from build123d import *

# Parameters (mm, degrees)
SKETCH1_W           = 160
SKETCH1_H           = 140
BOSS_EXTRUDE1_DEPTH = 16
SKETCH2_R           = 6.5
CUT_EXTRUDE1_DEPTH  = 11
SKETCH3_R           = 3
CUT_EXTRUDE2_DEPTH  = 214.20412754


with BuildPart() as part:
    # Sketch1 → Boss-Extrude1 (new body)
    with BuildSketch(Plane.XY):
        with Locations((-80, -70)):
            Rectangle(SKETCH1_W, SKETCH1_H)
    extrude(amount=BOSS_EXTRUDE1_DEPTH)

    # Sketch2 → Cut-Extrude1 (cut)
    with BuildSketch(Plane.XY.offset(16)):
        with Locations((-131.336336798, -99.63904787)):
            Circle(SKETCH2_R)
        with Locations((-80, -10.721904261)):
            Circle(SKETCH2_R)
        with Locations((-28.663663202, -99.63904787)):
            Circle(SKETCH2_R)
    extrude(amount=-CUT_EXTRUDE1_DEPTH, mode=Mode.SUBTRACT)

    # Sketch3 → Cut-Extrude2 (cut, through all)
    with BuildSketch(Plane.XY.offset(16)):
        with Locations((-18, -43)):
            Circle(SKETCH3_R)
        with Locations((-102, -43)):
            Circle(SKETCH3_R)
    extrude(amount=-CUT_EXTRUDE2_DEPTH, mode=Mode.SUBTRACT)


solid = part.part
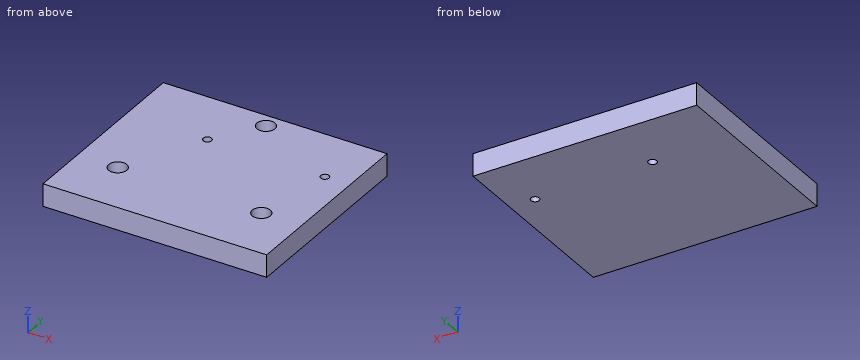
Design review of the part built by this model. Coordinates are the model's own, in mm. Round coordinates to 2 decimals unless told otherwise and drop trailing zeros. Write each loop counter-clockwise with the first axis right and the second up, starting at its lowest first coordinate (ties: lowest second). Pieces come first, ordered by that corner, then holes. Notation, with made-up numbers: (-13.5, 43) -> (40.5, 43) arc R6 ccw to (40.5, 53) -> close; hole circle Ø7 at (19.25, 6.25). An arc over 180 degrees is marked (long way). One line per item, written item: value. Start each with the question number.
Q1. Add section D-D (x = -80). Give the boundary of the cut face in (y, z), then the cut area to 3 significant figures.
Q2. Insertion check: P1, Ø2, axis at x = -52, y = -65.5, coming from the -Z side; P2, Ø3.5, axis at x = -102, y = -43, coming from the -Z side. Each pin has a flat end and moves straight along its axis. Give the tip position at first contact, or say it passes through.
Q3. Add section C-C (z = 9). Give the boundary of the cut face in (x, y).
Q4. To check wall thickness, follow probe 1 along X at (y, z) = (-10, 12); probe 2 along X at (y, z) = (-42, 2); probe 3 along Y at (x, z) = (-17, 4.25). State the ranges of each line that lie inside material, in increasing order.
Q5. Add section B-B (y = -43). Give the boundary of the cut face in (x, z).
Q6. Add section A-A (x = -102). Give the boundary of the cut face in (y, z), then the cut area to 3 significant figures.
Response:
1. outline: (-140, 0) -> (0, 0) -> (0, 16) -> (-4.22, 16) -> (-4.22, 5) -> (-17.22, 5) -> (-17.22, 16) -> (-140, 16) -> close
1. area: 2,100 mm^2
2. P1: stops at z = 0
2. P2: passes through
3. outline: (-160, -140) -> (0, -140) -> (0, 0) -> (-160, 0) -> close; hole circle Ø13 at (-131.34, -99.64); hole circle Ø6 at (-102, -43); hole circle Ø13 at (-80, -10.72); hole circle Ø13 at (-28.66, -99.64); hole circle Ø6 at (-18, -43)
4. probe 1: x = -160 to -86.46, -73.54 to 0
4. probe 2: x = -160 to -104.83, -99.17 to -20.83, -15.17 to 0
4. probe 3: y = -140 to -45.83, -40.17 to 0
5. outline: (-160, 0) -> (-105, 0) -> (-105, 16) -> (-160, 16) -> close; (-99, 0) -> (-21, 0) -> (-21, 16) -> (-99, 16) -> close; (-15, 0) -> (0, 0) -> (0, 16) -> (-15, 16) -> close
6. outline: (-140, 0) -> (-46, 0) -> (-46, 16) -> (-140, 16) -> close; (-40, 0) -> (0, 0) -> (0, 16) -> (-40, 16) -> close
6. area: 2,140 mm^2
